Could you check a few things on this drawing? It's one solid part, dimensions in mm from its lowest x, y, z. A direction names the side the tool comes from. Give positions to 0.01 mm unless a question says otherwise; leave off trailing zeros. Write each loop counter-clockwise with the first axis right and the second up, starting at its lowest first coordinate (ties: lowest second). Pieces come first, ordered by that corner, then holes.
1. On a 3-axis mill with a long thin cutter (end or side, diameter ignored), from which of +Z, -Z, +X, -X, +Y, -Y can I reach the whole of each face in a straight line? I mean the marked faces 1, 2, 3 and 4. Say none if no direction works.
2. I'm going to push flat-ended pins straight in: pin 1 (5 mm diameter, centred on x = 28, y = 5.5, fed in from +Z); pin 2 (1.1 mm diameter, centred on y = 5, z = 43.5, fed in from +X); pin 3 (1.5 mm diameter, centred on x = 7.5, y = 3, fed in from +Z). Where does each tip first touch, or does it pass through?
3. Thinking about a two-plate mould opening in X: for the marked faces 5, 6, 7 and 8, which applies, pulls with the +X half, pulls with the -X half, needs draft (parallel to the pull), parting line crosses it, or undercut?
4. Suppose I cut it at C-C (x = 4.5). Please give me the cut outline in (y, z).
5. Suppose I cut it at B-B (y = 4). Please give me the cut outline in (x, z).
6. If I drill on probe 1 along X at (y, z) = (2, 39); probe 2 along Z at (x, y) = (2.75, 7); probe 3 along Z at (x, y) = (22.5, 7), over which ranges is the centre line in solid material (lowest first)?
7. Suppose I cut it at A-A (z = 5). Please give me the cut outline in (x, y).
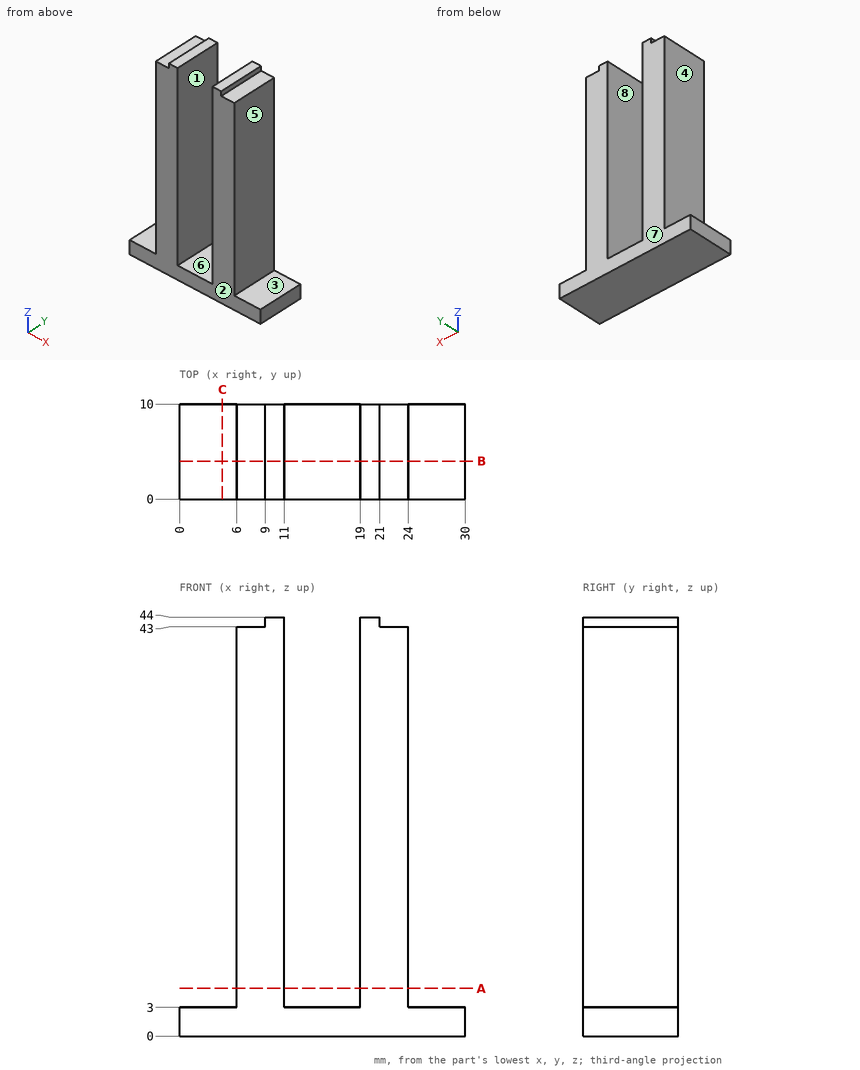
Checks:
1. face 1: +Z, +Y, -Y
1. face 2: +Z, -Z, +X, -X, -Y
1. face 3: +Z, +X, +Y, -Y
1. face 4: +Z, -X, +Y, -Y
2. pin 1: stops at z = 3
2. pin 2: stops at x = 24
2. pin 3: stops at z = 43
3. face 5: pulls with the +X half
3. face 6: undercut
3. face 7: needs draft
3. face 8: undercut
4. outline: (0, 0) - (10, 0) - (10, 3) - (0, 3) - close
5. outline: (0, 0) - (30, 0) - (30, 3) - (24, 3) - (24, 43) - (21, 43) - (21, 44) - (19, 44) - (19, 3) - (11, 3) - (11, 44) - (9, 44) - (9, 43) - (6, 43) - (6, 3) - (0, 3) - close
6. probe 1: x = 6 to 11, 19 to 24
6. probe 2: z = 0 to 3
6. probe 3: z = 0 to 43
7. outline: (6, 0) - (11, 0) - (11, 10) - (6, 10) - close; (19, 0) - (24, 0) - (24, 10) - (19, 10) - close
